from build123d import *

# Parameters (mm, degrees)
F1_DEPTH = 8
F2_R     = 2.5
F3_R     = 5
F4_DEPTH = 5
F5_R     = 5
F6_DEPTH = 5


# Not quite as in the source:
# - a feature names something its author has since deleted; it is built from what else it names


with BuildPart() as f1:
    # F0 (on Front) → F1 (new body)
    with BuildSketch(Plane.XZ):
        with BuildLine():
            ThreePointArc((0, -7.5), (-7.5, 0), (0, 7.5))
            Line((0, 7.5), (-153.126, 7.5))
            Line((-153.126, 7.5), (-153.126, -7.5))
            Line((-153.126, -7.5), (0, -7.5))
        make_face()
        with BuildLine():
            Line((0, 5), (0, 7.5))
            ThreePointArc((0, 7.5), (-7.5, 0), (0, -7.5))
            Line((0, -7.5), (0, -5))
            ThreePointArc((0, -5), (-5, 0), (0, 5))
        make_face()
        with BuildLine():
            ThreePointArc((0, -7.5), (5.3033008589, -5.3033008589), (7.5, 0))
            ThreePointArc((7.5, 0), (5.3033008589, 5.3033008589), (0, 7.5))
            Line((0, 7.5), (0, 5))
            ThreePointArc((0, 5), (3.5355339059, 3.5355339059), (5, 0))
            ThreePointArc((5, 0), (3.5355339059, -3.5355339059), (0, -5))
            Line((0, -5), (0, -7.5))
        make_face()
    extrude(amount=F1_DEPTH)

    # F2
    f2_edges = [f1.edges().sort_by_distance(p)[0] for p in [
        (-153.126, -4, 7.5),
        (-153.126, -4, -7.5),
    ]]
    fillet(f2_edges, radius=F2_R)

    # F3 (on face) → F4 (join)
    with BuildSketch(Plane(origin=(0, 0, 0), x_dir=(-1, 0, 0), z_dir=(0, 1, 0))):
        with Locations((145.626, 0)):
            Circle(F3_R)
    extrude(amount=F4_DEPTH)

    # F5 (on face) → F6 (cut)
    with BuildSketch(Plane.XZ.offset(8)):
        with Locations((-145.626, 0)):
            Circle(F5_R)
    extrude(amount=-F6_DEPTH, mode=Mode.SUBTRACT)


solid = f1.part
Geometry: final body of the model. Coordinates: model frame, mm. A direction names the side the tool comes from. Coordinates: 2 decimals unless noted, no trailing zeros. Order: outer loops, then holes, each group sorted by start corner. A loop starts at its lowest first (then second) coordinate and runs counter-clockwise, first axis right, second up.
(1) Material intervals for probe 1 along Z at (x, y) = (-0.5, -0.5); probe 2 along Y at (x, z) = (-75, -2); probe 3 along X at (y, z) = (4.75, 0.25), sorted ascending.
(2) Section query A-A (z = 2.5). Return the cut outline in (x, y).
(3) Section query B-B (x = -65). Return the cut outline in (y, z), plus the area to 3 significant figures.
(4) First-contact query: pin 1 (7.5 mm diameter, centred on x = -88.5, z = 0.5, fed in from +Y); pin 2 (3 mm diameter, centred on x = -147.5, z = 0.5, fed in from -Y). Flat tips, straight axial feed; report the tip coordinate or a pass-through.
(5) Access query for faces 4 (the face through (-74, -8, 0)), 5 (the face through (-146, -3, 0)), 6 (the face through (-150.395, 2.465, 1.502)). Directions: +Z, -Z, +X, -X, +Y, -Y. A direction counts if a zero-diameter tool reaches every point of the face in a straight line with its end or side. Return the directions, or none.
(6) Section query C-C (y = 3). Return the cut outline in (x, z), plus the area to 3 significant figures.
(7) Draft query along Z for faces 1 (the face through (-150.62, -5.54, 0.22)), 2 (the face through (-152.41, -4.06, -6.75)), 3 (the face through (-152.37, -4.06, 6.79)). Return one class per face: pulls with the +Z half, pulls with the -Z half, needs draft (parallel to the pull), parting line crosses it, or undercut.
Solution:
1. probe 1: z = -7.5 to -4.97, 4.97 to 7.5
1. probe 2: y = -8 to 0
1. probe 3: x = -150.62 to -140.63
2. outline: (-153.13, -8) - (-149.96, -8) - (-149.96, -3) - (-141.3, -3) - (-141.3, -8) - (-4.33, -8) - (-4.33, 0) - (-141.3, 0) - (-141.3, 5) - (-149.96, 5) - (-149.96, 0) - (-153.13, 0) - close; (4.33, -8) - (7.07, -8) - (7.07, 0) - (4.33, 0) - close
3. outline: (-8, -7.5) - (0, -7.5) - (0, 7.5) - (-8, 7.5) - close
3. area: 120 mm2
4. pin 1: stops at y = 0
4. pin 2: stops at y = -3
5. face 4: +Z, -Z, +X, -X, -Y
5. face 5: -Y
5. face 6: +Y
6. outline: circle Ø10 at (-145.63, 0)
6. area: 78.5 mm2
7. face 1: undercut
7. face 2: pulls with the -Z half
7. face 3: pulls with the +Z half
